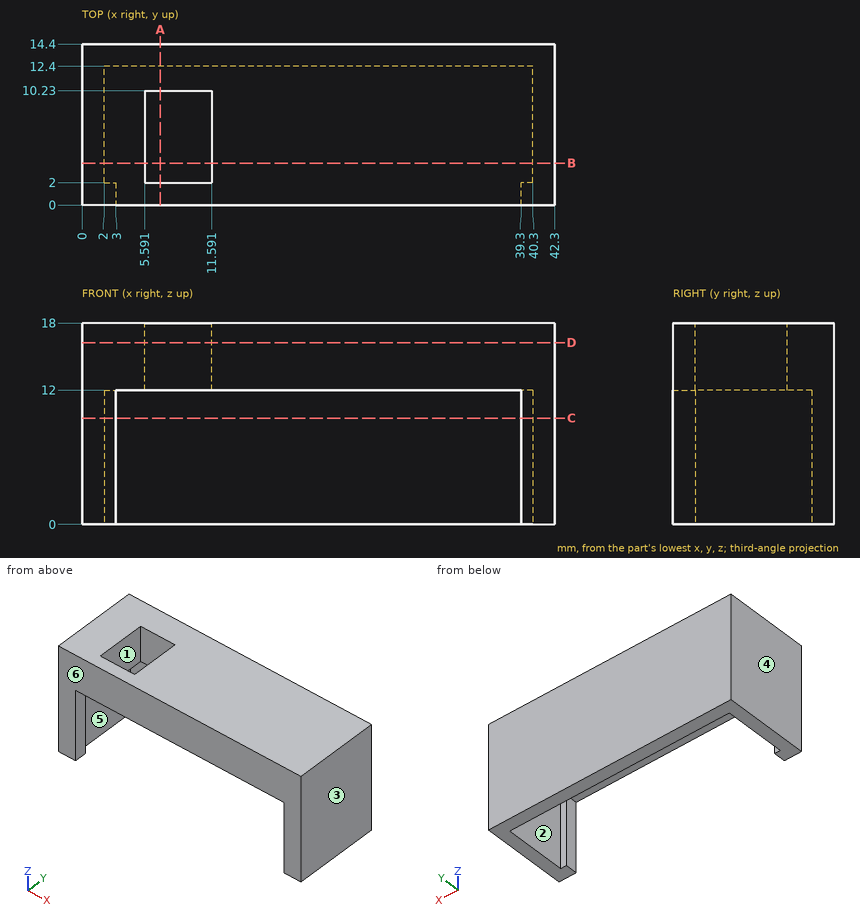
Source: three-view drawing plus pictorial views. Frame: mm from the lowest corner of the part. A direction names the side the tool comes from. Round coordinates to 2 decimals unless told otherwise and drop trailing zeros. Loops run counter-clockwise (first coordinate to the right, second up) from the corner with the lowest first, then second, coordinate; pieces in that order, holes last. Notation, with made-up numbers: M -16.75,83 L 19.25,83 A12 ccw 19.25,105 Z; hole C 13.25,-14 d2. An arc over 180 degrees is marked long. Put each result on its own line as item: value.
(1) Section C-C, the plane z = 9.5. Return loops of the section in (x, y), and give its area (3 significant figures).
Solutions:
outline: M 0,0 L 3,0 L 3,2 L 2,2 L 2,12.4 L 40.3,12.4 L 40.3,2 L 39.3,2 L 39.3,0 L 42.3,0 L 42.3,14.4 L 0,14.4 Z
area: 138 mm²
(2) Pull-direction query (Y, two-part tool) for the marked faces 4, 5 and 6; classes: released by +Y, released by -Y, zero draft, split by the parting line, or undercut.
Solutions:
face 4: zero draft
face 5: undercut
face 6: released by -Y
(3) First-contact query: pin 1 (6 mm diameter, centred on x = 16, z = 4, fed in from -Y). Flat tip, straight axial feed; report the tip coordinate or a pass-through.
Solutions:
pin 1: y = 12.4
(4) Ray query, line 1 (X direction, y = 9.75, z = 8.25); line 2 (X direction, y = 9.5, z = 17); line 3 (Y direction, x = 34.5, z = 2). Return the intervals inside material, ascending. Write a range as [from, to].
Solutions:
line 1: [0, 2], [40.3, 42.3]
line 2: [0, 5.59], [11.59, 42.3]
line 3: [12.4, 14.4]
(5) Access query for the marked faces 1, 2 and 3. Directions: +Z, -Z, +X, -X, +Y, -Y. A direction counts if a zero-diameter tool reaches every point of the face in a straight line with its end or side. Return the directions, or none.
Solutions:
face 1: +Z, -Z
face 2: -Z
face 3: +Z, -Z, +X, +Y, -Y
(6) Section D-D, the plane z = 16.25. Return loops of the section in (x, y), and give its area (3 significant figures).
Solutions:
outline: M 0,0 L 42.3,0 L 42.3,14.4 L 0,14.4 Z; hole M 5.59,2 L 11.59,2 L 11.59,10.23 L 5.59,10.23 Z
area: 560 mm²
(7) Section A-A, the plane x = 7. Return loops of the section in (y, z), and give its area (3 significant figures).
Solutions:
outline: M 0,12 L 2,12 L 2,18 L 0,18 Z; M 10.23,12 L 12.4,12 L 12.4,0 L 14.4,0 L 14.4,18 L 10.23,18 Z
area: 61.0 mm²
(8) Section B-B, the plane y = 3.75. Return loops of the section in (x, z), and give its area (3 significant figures).
Solutions:
outline: M 0,0 L 2,0 L 2,12 L 5.59,12 L 5.59,18 L 0,18 Z; M 11.59,12 L 40.3,12 L 40.3,0 L 42.3,0 L 42.3,18 L 11.59,18 Z
area: 266 mm²
